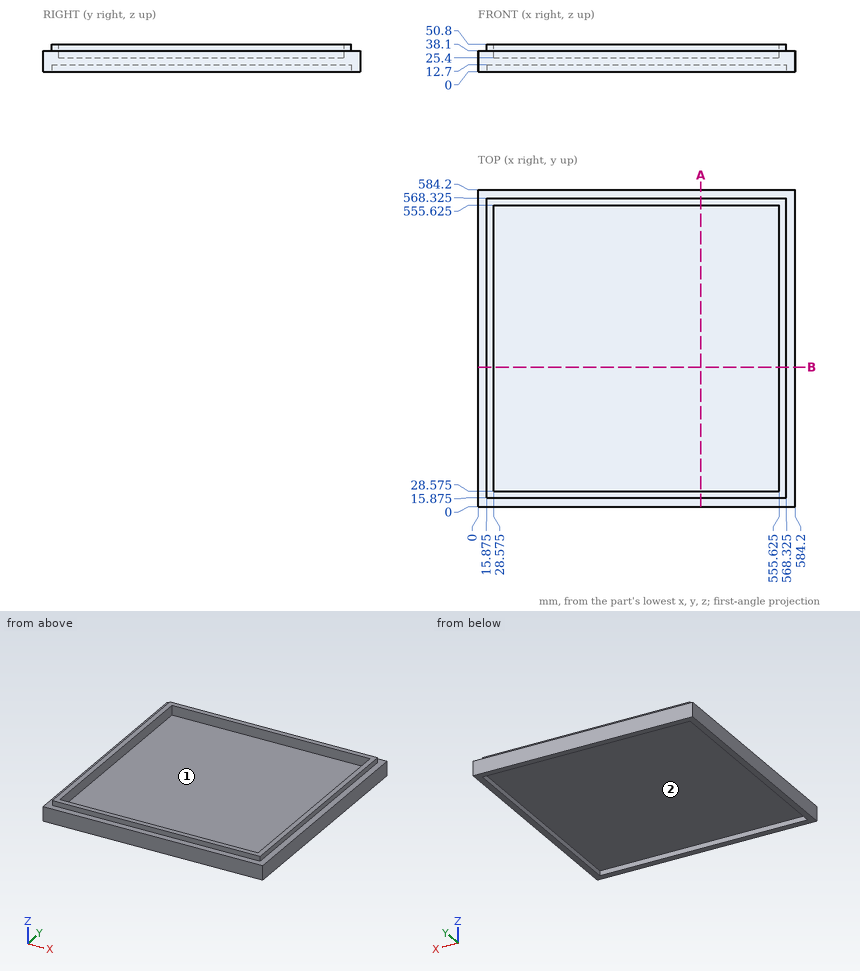
For this review, use the dimensioned drawing (mm, ordinates from the lowest corner) and the shaded views. A direction names the side the tool comes from. Give positions to 0.01 mm unless a question says otherwise; leave off trailing zeros. Write each loop counter-clockwise with the first axis right and the second up, starting at its lowest first coordinate (ties: lowest second). Pieces come first, ordered by that corner, then holes.
(1) For P1, Ø4, axis at x = 306.5, y = 332.5, coming from the -Z side; P2, Ø4, axis at x = 192.5, z = 41.5, coming from the -Y side (3 decimals); P3, Ø6.5, axis at y = 427.5, z = 44.5, coming from the -X side (3 decimals), all flat-tipped, find the tip position at first contact; note any pin that passes through.
(2) To check wall thickness, follow L1, parallel to Y at x = 446, z = 28.5 (3 decimals); L2, parallel to X at y = 296, z = 39 (3 decimals); L3, parallel to Y at x = 128.5, z = 7.5 (3 decimals). State the ranges of each line that lie inside material, in increasing order.
(3) Tool access review of the marked faces 1 and 2: name each direction out of +Z, -Z, +X, -X, +Y, -Y from which nothing blocks a thin tool from reaching the whole face with its end or side.
(4) Consider section A-A, the plane x = 410.5. Give the boundary of the cut face in (y, z) (3 decimals).
Returned:
1. P1: stops at z = 12.7
1. P2: stops at y = 15.875
1. P3: stops at x = 15.875
2. L1: y = 0 to 28.575, 555.625 to 584.2
2. L2: x = 15.875 to 28.575, 555.625 to 568.325
2. L3: y = 0 to 15.875, 568.325 to 584.2
3. face 1: +Z
3. face 2: -Z
4. outline: (0, 0) - (15.875, 0) - (15.875, 12.7) - (568.325, 12.7) - (568.325, 0) - (584.2, 0) - (584.2, 38.1) - (568.325, 38.1) - (568.325, 50.8) - (555.625, 50.8) - (555.625, 25.4) - (28.575, 25.4) - (28.575, 50.8) - (15.875, 50.8) - (15.875, 38.1) - (0, 38.1) - close
